Build history of the part. All positions in model axes, mm. A direction names the side the tool comes from. Round coordinates to 2 decimals unless told otherwise and drop trailing zeros. Order: outer loops, then holes, each group sorted by start corner. A loop starts at its lowest first (then second) coordinate and runs counter-clockwise, first axis right, second up. Notation, with made-up numbers: (-36.5, 12.25) -> (-20.5, 12.25) arc R23 ccw to (-20.5, 48.25) -> close; hole circle Ø2 at (15.25, 61). An arc over 180 degrees is marked (long way). Write item = value, one per line.
Autodesk Inventor part; units mm, degrees
ref_plane "YZ Plane" through (0, 0, 0) normal (1, 0, 0) x (0, 1, 0)
ref_plane "XZ Plane" through (0, 0, 0) normal (0, 1, 0) x (-1, 0, 0)
ref_plane "XY Plane" through (0, 0, 0) normal (0, 0, 1) x (1, 0, 0)
sketch "Sketch1" plane through (0, 0, 0) normal (0, 0, 1) x (1, 0, 0)
  circle A0 centre (0, 0) radius 24.892
  circle A1 centre (267.462, 0) radius 24.892
  line L0 (0, 0) -> (267.462, 0) construction
  line L1 (0, -25.019) -> (267.462, -25.019)
  line L2 (267.462, 25.019) -> (0, 25.019)
  arc A2 (0, 25.019) -> (0, -25.019) centre (0, 0) ccw
  arc A3 (267.462, -25.019) -> (267.462, 25.019) centre (267.462, 0) ccw
  line L3 (0, 28.194) -> (267.462, 28.194)
  arc A4 (267.462, -28.194) -> (267.462, 28.194) centre (267.462, 0) ccw
  line L4 (267.462, -28.194) -> (0, -28.194)
  arc A5 (0, 28.194) -> (0, -28.194) centre (0, 0) ccw
  line L5 (7.3323, 0) -> (3.6662, -6.35)
  line L6 (3.6662, -6.35) -> (-3.6662, -6.35)
  line L7 (-3.6662, -6.35) -> (-7.3323, 0)
  line L8 (-7.3323, 0) -> (-3.6662, 6.35)
  line L9 (-3.6662, 6.35) -> (3.6662, 6.35)
  line L10 (3.6662, 6.35) -> (7.3323, 0)
  line L11 (274.7943, 0) -> (271.1282, -6.35)
  line L12 (271.1282, -6.35) -> (263.7958, -6.35)
  line L13 (263.7958, -6.35) -> (260.1297, 0)
  line L14 (260.1297, 0) -> (263.7958, 6.35)
  line L15 (263.7958, 6.35) -> (271.1282, 6.35)
  line L16 (271.1282, 6.35) -> (274.7943, 0)
  point P0 (133.731, 0)
  dimension "d0" = 49.784
  dimension "d1" = 267.462
  dimension "d2" = 3.175
  dimension "d3" = 0.127
  dimension "d8" = 12.7
extrude "Extrusion2" add sketch "Sketch1" along normal blind 9 contours L3 A4 L4 A5
properties part number "DGB_005_Short Belt_Gates_695-5M-09"
Q1. Cut at A-A, the plane y = 0. List the corners of the cut face in (x, z), and give its area (4 significant figures).
Check values:
outline = (-28.19, 0) -> (-25.02, 0) -> (-25.02, 9) -> (-28.19, 9) -> close; (292.48, 0) -> (295.66, 0) -> (295.66, 9) -> (292.48, 9) -> close
area = 57.15 mm²
Q2. Flat gauge pins, fed straight in: pin 1 (8 mm diameter, centred on x = 185.5, y = -21.5, fed in from +Z); pin 2 (3 mm diameter, centred on y = -5.5, z = 4, fed in from -X); pin 3 (5 mm diameter, centred on y = 11, z = 2.5, fed in from -X); pin 4 (3 mm diameter, centred on y = 5.5, z = 6.5, fed in from +X). Where does each tip first touch, or does it go through?
Check values:
pin_1 = 9
pin_2 = -27.91
pin_3 = -26.88
pin_4 = 295.37
Q3. Cut at B-B, the plane x = 46. List the corners of the cut face in (y, z).
Check values:
outline = (-28.19, 0) -> (-25.02, 0) -> (-25.02, 9) -> (-28.19, 9) -> close; (25.02, 0) -> (28.19, 0) -> (28.19, 9) -> (25.02, 9) -> close
Q4. Probe probe 1 along Y at (x, z) = (141.5, 2); probe 2 along X at (y, z) = (-11, 5.5); probe 3 along X at (y, z) = (20, 2.25). List the from-to ranges inside material, lowest first.
Check values:
probe_1 = -28.19 to -25.02, 25.02 to 28.19
probe_2 = -25.96 to -22.47, 289.93 to 293.42
probe_3 = -19.87 to -15.03, 282.49 to 287.33
Q5. Cut at C-C, the plane z = 4.75. List the corners of the cut face in (x, y).
Check values:
outline = (0, -28.19) -> (267.46, -28.19) arc R28.19 ccw to (267.46, 28.19) -> (0, 28.19) arc R28.19 ccw to start; hole (0, -25.02) -> (267.46, -25.02) arc R25.02 ccw to (267.46, 25.02) -> (0, 25.02) arc R25.02 ccw to start
Q6. Mould opens along X. For faces 3 (the face through (121, 25.2, 9)), 4 (the face through (132, -25.019, 4)), 5 (the face through (-28.187, -0.62, 4.437)) say: released by +X, released by -X, zero draft, split by the parting line, or undercut.
Check values:
face_3 = zero draft
face_4 = undercut
face_5 = released by -X
Q7. Which spindle directions (+Z, -Z, +X, -X, +Y, -Y) get a long thin tool onto all of the face, cutting with end or side? Do faces 1 (the face through (136, 25.019, 4)), 2 (the face through (121, 25.2, 0)). Say none if no direction does.
Check values:
face_1 = +Z, -Z
face_2 = -Z, +X, -X, +Y, -Y
